The listing builds one solid part. Answer for the finished solid, in the listing's coordinates (mm). A direction names the side the tool comes from. Coordinates: 2 decimals unless noted, no trailing zeros. Order: outer loops, then holes, each group sorted by start corner. A loop starts at its lowest first (then second) coordinate and runs counter-clockwise, first axis right, second up. Notation, with made-up numbers: (3.5, 57.5) - (37.5, 57.5) arc R35 ccw to (37.5, 89.5) - close; hole circle Ø5 at (53.25, 68). An arc over 180 degrees is marked (long way). Use a Markdown table: item, result. Add a question column.
Item 1: Flat-ended cylindrical pins translate along their axes: P1, Ø4, axis at x = 0, y = 34.5, coming from the +Z side; P2, Ø2, axis at y = 24, z = 14.5, coming from the -X side; P3, Ø5, axis at x = 35, z = 10, coming from the -Y side. Find the tip coordinate at first contact, or state that the pin passes through.
Item 2: The part is cut by section C-C, the plane x = 17. Give the vertices of the cut face in (y, z).
Item 3: The part is cut by section B-B, the plane y = 15.5. Give the vertices of the cut face in (x, z), then the cut area to 3 significant figures.
Item 4: The part is cut by section A-A, the plane x = 0. Give the vertices of the cut face in (y, z) (3 decimals).
Item 5: Find the intervals of material crossed by line 1 along Y through (x, z) = (0, 20.5) (3 decimals); line 2 along Y through (x, z) = (-3, 4); line 3 along X through (y, z) = (-5, 0.5), in increasing order.
Item 6: The mould has two halves that part along Y. Classify faces 4 (the flat face through (17, 25, -2)), 5 (the cylindrical face through (29.97, -1.32, -0.99)): released by +Y, released by -Y, zero draft, split by the parting line, or undercut.
Item 7: For faces 1 (the flat face through (34, 2.4, 14)), 2 (the flat face through (30, -17, 19.9)), 3 (the flat face through (-20, -25, 22)), determine the directions among +Z, -Z, +X, -X, +Y, -Y from which every point of the face is accessible in a straight line to the end or side of a thin tool.
Item 8: The part is cut by section D-D, the plane y = -17.25. Give the vertices of the cut face in (x, z).
Autodesk Inventor part; units mm, degrees
ref_plane "YZ Plane" through (0, 0, 0) normal (1, 0, 0) x (0, 1, 0)
ref_plane "XZ Plane" through (0, 0, 0) normal (0, 1, 0) x (-1, 0, 0)
ref_plane "XY Plane" through (0, 0, 0) normal (0, 0, 1) x (1, 0, 0)
sketch "Skizze1" plane through (0, 0, 0) normal (0, 0, 1) x (1, 0, 0)
  circle A0 centre (0, 0) radius 31.5
  circle A1 centre (0, 0) radius 37.5
  dimension "d0" = 63
  dimension "d1" = 75
extrude "Extrusion1" add sketch "Skizze1" along normal blind 22
sketch "Skizze2" plane through (0, 0, 0) normal (0, 0, -1) x (-1, 0, 0)
  circle A0 centre (0, 0) radius 37.5
  circle A1 centre (0, 0) radius 30
  dimension "d4" = 75
  dimension "d5" = 60
extrude "Extrusion2" add sketch "Skizze2" along normal blind 2
sketch "Skizze3" plane through (0, 0, 22) normal (0, 0, 1) x (1, 0, 0)
  point P0 (0, 0)
  point P1 (0, 34.5)
  dimension "d8" = 34.5
hole "Bohrung1" at (0, 34.5, 22) direction (0, 0, -1) diameter 5.05 depth 2.1
pattern_circular "Runde Anordnung1" count 3 over 360 about axis through (0, 0, 0) along (0, 0, 1) of "Bohrung1"
sketch "Skizze4" plane through (0, 0, 22) normal (0, 0, 1) x (1, 0, 0)
  line L0 (14.3077, 2.4) -> (40, 2.4)
  line L1 (40, 2.4) -> (40, -2.4)
  line L2 (40, -2.4) -> (14.3077, -2.4)
  line L3 (14.3077, -2.4) -> (14.3077, 2.4)
  point P0 (0, 0)
  dimension "d19" = 4.8
  dimension "d20" = 2.4
  dimension "d21" = 40
extrude "Extrusion3" cut sketch "Skizze4" against normal blind 18
fillet "Rundung1" radius 2 2 edges at (34.4158, 2.4, 4) (34.4158, -2.4, 4)
sketch "Skizze5" plane through (0, 0, 22) normal (0, 0, 1) x (1, 0, 0)
  point P0 (0, 0)
properties part number "Sensor63Deckel"
Solution:
| question | item | result |
|---|---|---|
| 1 | P1 | stops at z = 19.9 |
| 1 | P2 | stops at x = -29.62 |
| 1 | P3 | stops at y = -18.71 |
| 2 | outline | (-33.43, -2) - (-24.72, -2) - (-24.72, 0) - (-26.52, 0) - (-26.52, 22) - (-33.43, 22) - close; (24.72, -2) - (33.43, -2) - (33.43, 22) - (26.52, 22) - (26.52, 0) - (24.72, 0) - close |
| 3 | outline | (-34.15, -2) - (-25.69, -2) - (-25.69, 0) - (-27.42, 0) - (-27.42, 22) - (-34.15, 22) - close; (25.69, -2) - (34.15, -2) - (34.15, 22) - (27.42, 22) - (27.42, 0) - (25.69, 0) - close |
| 3 | area | 330 mm2 |
| 4 | outline | (-37.5, -2) - (-30, -2) - (-30, 0) - (-31.5, 0) - (-31.5, 22) - (-37.5, 22) - close; (30, -2) - (37.5, -2) - (37.5, 22) - (37.025, 22) - (37.025, 19.9) - (31.975, 19.9) - (31.975, 22) - (31.5, 22) - (31.5, 0) - (30, 0) - close |
| 5 | line 1 | y = -37.5 to -31.5, 31.5 to 31.975, 37.025 to 37.5 |
| 5 | line 2 | y = -37.38 to -31.36, 31.36 to 37.38 |
| 5 | line 3 | x = -37.17 to -31.1, 31.1 to 37.17 |
| 6 | face 4 | zero draft |
| 6 | face 5 | undercut |
| 7 | face 1 | +Z, +X |
| 7 | face 2 | +Z |
| 7 | face 3 | +Z, +X, -X, +Y, -Y |
| 8 | outline | (-33.3, -2) - (-24.54, -2) - (-24.54, 0) - (-26.36, 0) - (-26.36, 22) - (-27.35, 22) - (-27.35, 19.9) - (-32.4, 19.9) - (-32.4, 22) - (-33.3, 22) - close; (24.54, -2) - (33.3, -2) - (33.3, 22) - (32.4, 22) - (32.4, 19.9) - (27.35, 19.9) - (27.35, 22) - (26.36, 22) - (26.36, 0) - (24.54, 0) - close |
